from build123d import *

# Parameters (mm, degrees)
BOSS_EXTRUDE1_DEPTH = 25.4
SKETCH3_W           = 39.775281732
SKETCH3_H           = 6.35
BOSS_EXTRUDE2_DEPTH = 2.54
SKETCH4_W           = 3.175
SKETCH4_H           = 56.314123931
CUT_EXTRUDE1_DEPTH  = 0.254


with BuildPart() as part:
    # Sketch1 → Boss-Extrude1 (new body)
    with BuildSketch(Plane.XY):
        Polygon((0, 0), (16.712640866, 0), (23.062640866, 0), (39.775281732, 0), (39.775281732, 39.8648657), align=None)
    extrude(amount=BOSS_EXTRUDE1_DEPTH)

    # Sketch3 → Boss-Extrude2 (add)
    with BuildSketch(Plane.XZ):
        with Locations((19.887640866, 12.7)):
            Rectangle(SKETCH3_W, SKETCH3_H)
    extrude(amount=BOSS_EXTRUDE2_DEPTH)

    # Sketch4 → Cut-Extrude1 (cut)
    with BuildSketch(Plane(origin=(0, 0, 0), x_dir=(0, 0, 1), z_dir=(-0.7079017290339694, 0.706310938631646, 0))):
        with Locations((12.7, 28.157061966)):
            Rectangle(SKETCH4_W, SKETCH4_H)
    extrude(amount=-CUT_EXTRUDE1_DEPTH, mode=Mode.SUBTRACT)


solid = part.part
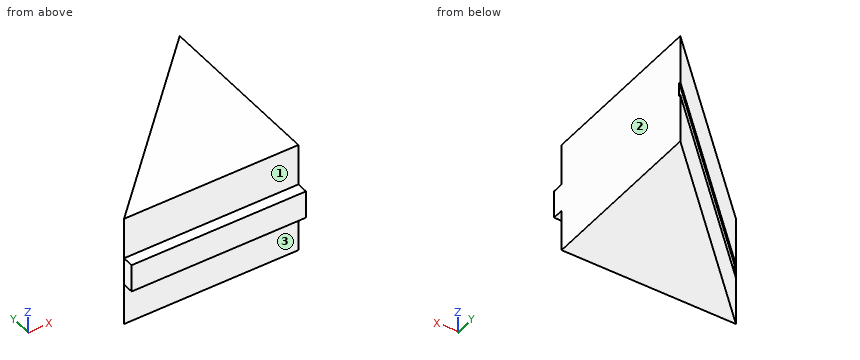
Here's how the part is built. I have some questions about the finished solid (model axes, mm). Face numbers are marked on the shaded views. A direction names the side the tool comes from. Give positions to 0.01 mm unless a question says otherwise; leave off trailing zeros. Write each loop counter-clockwise with the first axis right and the second up, starting at its lowest first coordinate (ties: lowest second). Pieces come first, ordered by that corner, then holes. Notation, with made-up numbers: (43.25, -12) -> (87.25, -12) arc R18 ccw to (87.25, 21) -> close; hole circle Ø6 at (52, -33.5). An arc over 180 degrees is marked (long way). Use one line per item in the form item = value. Start each with the question number.
1. Imagine slicing it at A-A on y = 2.5. List the corners of the cut face in (x, z) for me.
2. Imagine slicing it at C-C on z = 1.75. List the corners of the cut face in (x, y) for me, plus the area to 3 significant figures.
3. Will these pins go through, and if not, where does the flat tip stop? pin 1 Ø2 at (x, y) = (13, -1.5) entering from +Z (3 decimals); pin 2 Ø3 at (y, z) = (23.5, 19.5) entering from -X; pin 3 Ø8 at (y, z) = (19, 9.5) entering from -X.
4. If I drill on L1, parallel to X at y = 10, z = 5; L2, parallel to Y at x = 13.5, z = 14.5; L3, parallel to Y at x = 15.5, z = 11.5, over which ranges is the centre line in solid material (lowest first)?
5. On a 3-axis mill with a long thin cutter (end or side, diameter ignored), from which of +Z, -Z, +X, -X, +Y, -Y can I reach the whole of each face in a straight line? I mean the marked faces 1, 2 and 3. Say none if no direction works.
Entries:
q1.outline = (2.49, 0) -> (39.78, 0) -> (39.78, 25.4) -> (2.49, 25.4) -> (2.49, 14.29) -> (2.85, 14.29) -> (2.85, 11.11) -> (2.49, 11.11) -> close
q2.outline = (0, 0) -> (39.78, 0) -> (39.78, 39.86) -> close
q2.area = 793 mm²
q3.pin_1 = 15.875
q3.pin_2 = 21.95
q3.pin_3 = 14.97
q4.L1 = 9.98 to 39.78
q4.L2 = -2.54 to 13.53
q4.L3 = -2.54 to 15.18
q5.face_1 = +Z, +X, -X, -Y
q5.face_2 = +Z, -Z, +X, +Y, -Y
q5.face_3 = -Z, +X, -X, -Y
